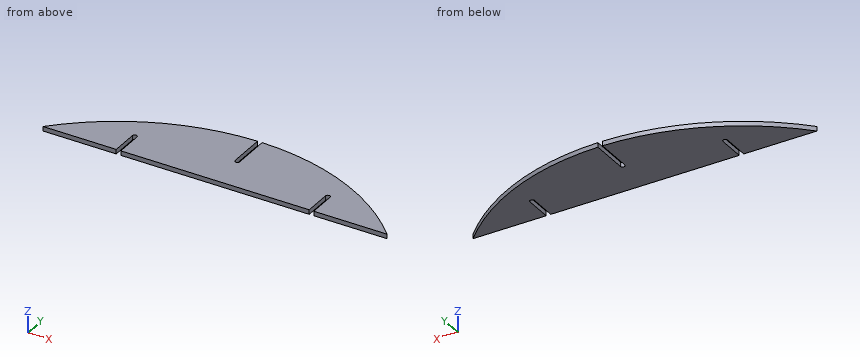
from build123d import *

# Parameters (mm, degrees)
F1_DEPTH = 12


with BuildPart() as f1:
    # F0 (on Top) → F1 (new body)
    with BuildSketch(Plane.XY):
        with BuildLine():
            Line((715.515126, 0), (909.030253, 0))
            ThreePointArc((909.030253, 0), (704.754458, 143.717449), (460.515126, 195.971199))
            Line((460.515126, 195.971199), (460.515126, 98))
            ThreePointArc((460.515126, 98), (454.515126, 92), (448.515126, 98))
            Line((448.515126, 98), (448.515126, 195.971199))
            ThreePointArc((448.515126, 195.971199), (204.275795, 143.717449), (0, 0))
            Line((0, 0), (193.515126, 0))
            Line((193.515126, 0), (193.515126, 71))
            ThreePointArc((193.515126, 71), (199.515126, 77), (205.515126, 71))
            Line((205.515126, 71), (205.515126, 0))
            Line((205.515126, 0), (703.515126, 0))
            Line((703.515126, 0), (703.515126, 71))
            ThreePointArc((703.515126, 71), (709.515126, 77), (715.515126, 71))
            Line((715.515126, 71), (715.515126, 0))
        make_face()
    extrude(amount=F1_DEPTH)


solid = f1.part
CAD build for the part. Positions are in the model's coordinates, mm. Round coordinates to 2 decimals unless told otherwise and drop trailing zeros. Order: outer loops, then holes, each group sorted by start corner. A loop starts at its lowest first (then second) coordinate and runs counter-clockwise, first axis right, second up. Notation, with made-up numbers: (25, 32.5) - (49, 32.5) arc R30 ccw to (49, 67.5) - close; hole circle Ø7 at (20.25, 33). An arc over 180 degrees is marked (long way). Return JSON: item names as keys, results as strings.
(1) Wall check: probe 1 along X at (y, z) = (65.5, 11.25); probe 2 along X at (y, z) = (59, 10.25); probe 3 along X at (y, z) = (96.5, 7). Give the ranges that are in metal, low to high. Write a range as from..to.
Answer key:
{"probe 1": "x = 72.29..193.52, 205.52..703.52, 715.52..836.74", "probe 2": "x = 64.03..193.52, 205.52..703.52, 715.52..845", "probe 3": "x = 116.17..448.71, 460.32..792.86"}
(2) Cut at C-C (x = 263.5). Give the cut face in (y, z), then the cut area to 3 significant figures.
Answer key:
{"outline": "(0, 0) - (166.1, 0) - (166.1, 12) - (0, 12) - close", "area": "1,990 mm^2"}
(3) Pin check, flat tips, straight feed: pin 1 Ø6 at (x, z) = (589.5, 4.5) entering from +Y; pin 2 Ø6 at (y, z) = (27.5, 4.5) entering from +X. Stop position of each tip, or through.
Answer key:
{"pin 1": "stops at y = 181.91", "pin 2": "stops at x = 884.59"}
(4) Cut at B-B (x = 519). Give the cut face in (y, z).
Answer key:
{"outline": "(0, 0) - (192.66, 0) - (192.66, 12) - (0, 12) - close"}
(5) Cut at A-A (z = 4.25). Give the cut face in (x, y), then the cut area to 3 significant figures.
Answer key:
{"outline": "(0, 0) - (193.52, 0) - (193.52, 71) arc R6 cw to (205.52, 71) - (205.52, 0) - (703.52, 0) - (703.52, 71) arc R6 cw to (715.52, 71) - (715.52, 0) - (909.03, 0) arc R625 ccw to (460.52, 195.97) - (460.52, 98) arc R6 cw to (448.52, 98) - (448.52, 195.97) arc R625 ccw to start", "area": "120,000 mm^2"}
